Work out the finished part from the listing and answer in its coordinate system (mm). Face numbers are marked on the shaded views. A direction names the side the tool comes from. Coordinates: 2 decimals unless noted, no trailing zeros. Loops run counter-clockwise (first coordinate to the right, second up) from the corner with the lowest first, then second, coordinate; pieces in that order, holes last. Notation, with made-up numbers: (29, 24.25) -> (36, 24.25) arc R28 cw to (36, 54.25) -> close; hole circle Ø9 at (-36.75, 19). An arc over 180 degrees is marked (long way). Use a Markdown table: item, result.
from build123d import *

# Parameters (mm, degrees)
SKETCH1_W           = 28
SKETCH1_H           = 28
BOSS_EXTRUDE1_DEPTH = 45
SKETCH2_R           = 11.5
BOSS_EXTRUDE2_DEPTH = 2
SKETCH3_R           = 2.25
BOSS_EXTRUDE3_DEPTH = 20
FILLET1_R           = 2.5


with BuildPart() as part:
    # Sketch1 → Boss-Extrude1 (new body)
    with BuildSketch(Plane(origin=(0, 0, 0), x_dir=(1, 0, 0), z_dir=(0, 1, 0))):
        Rectangle(SKETCH1_W, SKETCH1_H)
    extrude(amount=BOSS_EXTRUDE1_DEPTH)

    # Sketch2 → Boss-Extrude2 (add)
    with BuildSketch(Plane(origin=(0, 45, 0), x_dir=(1, 0, 0), z_dir=(0, 1, 0))):
        with Locations(Location((0, 0, 0), (0, 0, 90))):
            Circle(SKETCH2_R)
    extrude(amount=BOSS_EXTRUDE2_DEPTH)

    # Sketch3 → Boss-Extrude3 (add)
    with BuildSketch(Plane(origin=(0, 45, 0), x_dir=(1, 0, 0), z_dir=(0, 1, 0))):
        with Locations(Location((0, 0, 0), (0, 0, 270))):
            Circle(SKETCH3_R)
    extrude(amount=BOSS_EXTRUDE3_DEPTH)

    # Fillet1
    fillet1_edges = [part.edges().sort_by_distance(p)[0] for p in [
        (-14, 22.5, -14),
        (14, 22.5, -14),
        (14, 22.5, 14),
        (-14, 22.5, 14),
    ]]
    fillet(fillet1_edges, radius=FILLET1_R)


solid = part.part
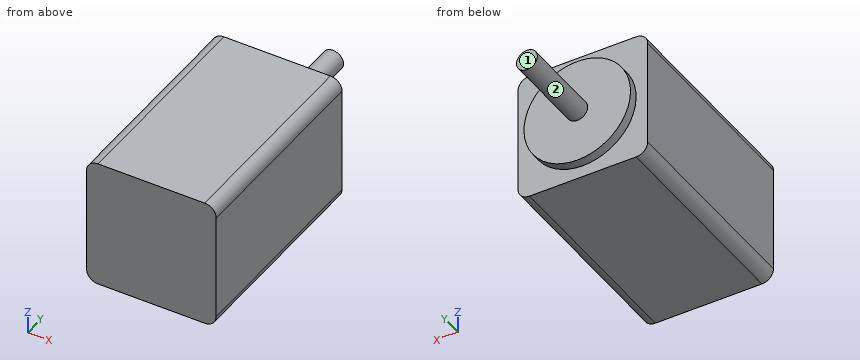
Q1. For the marked faces 1 and 2, determine the directions among +Z, -Z, +X, -X, +Y, -Y from which every point of the face is accessible in a straight line to the end or side of a thin tool.
Solved:
| item | result |
|---|---|
| face 1 | +Z, -Z, +X, -X, +Y |
| face 2 | +Y |
Q2. Consider line 1 (Z direction, x = 11.75, y = 18); line 2 (Y direction, x = 2.5, z = -11.5); line 3 (Y direction, x = -4, z = -10). Determine where each line is inside the solid, lowest interval first. Write a range as [from, to].
Solved:
| item | result |
|---|---|
| line 1 | [-13.99, 13.99] |
| line 2 | [0, 45] |
| line 3 | [0, 47] |
Q3. Section C-C on y = 57 is taken. Determine the outline of the cut face in (x, z).
Solved:
| item | result |
|---|---|
| outline | circle Ø4.5 at (0, 0) |
Q4. Given pin 1 Ø8 at (y, z) = (51.5, -2) entering from -X; pin 2 Ø4 at (x, z) = (0.5, 3.5) entering from -Y; pin 3 Ø1 at (x, z) = (-9, -6.5) entering from +Y, each flat-ended and moving along its own axis, determine where each tip first touches the part or whether it passes through.
Solved:
| item | result |
|---|---|
| pin 1 | x = -2.25 |
| pin 2 | y = 0 |
| pin 3 | y = 47 |
Q5. Section A-A on x = 0 is taken. Determine the outline of the cut face in (y, z), and give its area (3 significant figures).
Solved:
| item | result |
|---|---|
| outline | (0, -14) -> (45, -14) -> (45, -11.5) -> (47, -11.5) -> (47, -2.25) -> (65, -2.25) -> (65, 2.25) -> (47, 2.25) -> (47, 11.5) -> (45, 11.5) -> (45, 14) -> (0, 14) -> close |
| area | 1,390 mm² |
Q6. Section B-B on z = 0 is taken. Determine the outline of the cut face in (x, y), and give its area (3 significant figures).
Solved:
| item | result |
|---|---|
| outline | (-14, 0) -> (14, 0) -> (14, 45) -> (11.5, 45) -> (11.5, 47) -> (2.25, 47) -> (2.25, 65) -> (-2.25, 65) -> (-2.25, 47) -> (-11.5, 47) -> (-11.5, 45) -> (-14, 45) -> close |
| area | 1,390 mm² |
Q7. Section D-D on x = -8 is taken. Determine the outline of the cut face in (y, z), and give its area (3 significant figures).
Solved:
| item | result |
|---|---|
| outline | (0, -14) -> (45, -14) -> (45, -8.26) -> (47, -8.26) -> (47, 8.26) -> (45, 8.26) -> (45, 14) -> (0, 14) -> close |
| area | 1,290 mm² |
